Read the model definition and answer for the solid it produces. Units are mm, in the model's axes. A direction names the side the tool comes from. Coordinates: 2 decimals unless noted, no trailing zeros. Loops run counter-clockwise (first coordinate to the right, second up) from the corner with the lowest first, then second, coordinate; pieces in that order, holes last.
from build123d import *

# Parameters (mm, degrees)
F1_DEPTH = 29
F2_W     = 36
F2_H     = 11
F3_DEPTH = 127.001
F5_DEPTH = 58.001
F7_DEPTH = 58.001
F9_DEPTH = 33.001


with BuildPart() as f1:
    # F0 (on Front) → F1 (new body, symmetric)
    with BuildSketch(Plane.XZ):
        Polygon((11, 6), (11, 0), (116, 0), (116, 6), (127, 6), (127, 44), (0, 44), (0, 6), align=None)
    extrude(amount=F1_DEPTH, both=True)

    # F2 (on face) → F3 (cut, through all)
    with BuildSketch(Plane.YZ.offset(127)):
        with Locations((0, 38.5)):
            Rectangle(F2_W, F2_H)
    extrude(amount=-F3_DEPTH, mode=Mode.SUBTRACT)

    # F4 (on face) → F5 (cut, through all)
    with BuildSketch(Plane.XZ.offset(29)):
        with BuildLine():
            ThreePointArc((0, 15), (8.493903, 35.506097), (29, 44))
            Line((29, 44), (0, 44))
            Line((0, 44), (0, 15))
        make_face()
    extrude(amount=-F5_DEPTH, mode=Mode.SUBTRACT)

    # F6 (on face) → F7 (cut, through all)
    with BuildSketch(Plane.XZ.offset(29)):
        with BuildLine():
            ThreePointArc((98, 44), (118.506097, 35.506097), (127, 15))
            Line((127, 15), (127, 44))
            Line((127, 44), (98, 44))
        make_face()
    extrude(amount=-F7_DEPTH, mode=Mode.SUBTRACT)

    # F8 (on face) → F9 (cut, through all)
    with BuildSketch(Plane.XY.offset(33)):
        with BuildLine():
            Line((102, 4.898486), (83, 4.898486))
            ThreePointArc((83, 4.898486), (78.101514, 0), (83, -4.898486))
            Line((83, -4.898486), (102, -4.898486))
            ThreePointArc((102, -4.898486), (106.898486, 0), (102, 4.898486))
        make_face()
        with BuildLine():
            Line((44, 4.898486), (25, 4.898486))
            ThreePointArc((25, 4.898486), (20.101514, 0), (25, -4.898486))
            Line((25, -4.898486), (44, -4.898486))
            ThreePointArc((44, -4.898486), (48.898486, 0), (44, 4.898486))
        make_face()
    extrude(amount=-F9_DEPTH, mode=Mode.SUBTRACT)


solid = f1.part
Item 1: A cutting plane is placed at C-C on y = 0. Determine the outline of the cut face in (x, z).
Numbers:
outline: (0, 6) - (11, 6) - (11, 0) - (20.1, 0) - (20.1, 33) - (6.26, 33) arc R29 ccw to (0, 15) - close; (48.9, 0) - (78.1, 0) - (78.1, 33) - (48.9, 33) - close; (106.9, 0) - (116, 0) - (116, 6) - (127, 6) - (127, 15) arc R29 ccw to (120.74, 33) - (106.9, 33) - close
Item 2: A cutting plane is placed at D-D on y = 15.5. Determine the outline of the cut face in (x, z).
Numbers:
outline: (0, 6) - (11, 6) - (11, 0) - (116, 0) - (116, 6) - (127, 6) - (127, 15) arc R29 ccw to (120.74, 33) - (6.26, 33) arc R29 ccw to (0, 15) - close
Item 3: Which of the six approach directions +Z, -Z, +X, -X, +Y, -Y give full straight-line access (tool end or side, diameter ignored) to faces 4 (the face through (116, 0, 3)), 5 (the face through (64, -18, 38)), 6 (the face through (5, 0, 6)), 7 (the face through (92, -4.898, 17))?
Numbers:
face 4: -Z, +X, +Y, -Y
face 5: +Z, +X, -X
face 6: -Z, -X, +Y, -Y
face 7: +Z, -Z
Item 4: A cutting plane is placed at A-A on z = 12.5. Determine the outline of the cut face in (x, y), then the cut area to 3 significant figures.
Numbers:
outline: (0, -29) - (127, -29) - (127, 29) - (0, 29) - close; hole (25, -4.9) - (44, -4.9) arc R4.9 ccw to (44, 4.9) - (25, 4.9) arc R4.9 ccw to start; hole (83, -4.9) - (102, -4.9) arc R4.9 ccw to (102, 4.9) - (83, 4.9) arc R4.9 ccw to start
area: 6,840 mm2
Item 5: Given pin 1 (1 mm diameter, centred on y = -19, z = 34.5, fed in from +X); pin 2 (1 mm diameter, centred on y = 22, z = 28.5, fed in from -X); pin 3 (3.5 mm diameter, centred on x = 7.5, y = 1, fed in from -Z), each flat-ended and moving along its own axis, determine where each tip first touches the part or whether it passes through.
Numbers:
pin 1: stops at x = 119.91
pin 2: stops at x = 3.08
pin 3: stops at z = 6
Item 6: A cutting plane is placed at B-B on x = 96. Determine the outline of the cut face in (y, z).
Numbers:
outline: (-29, 0) - (-4.9, 0) - (-4.9, 33) - (-18, 33) - (-18, 44) - (-29, 44) - close; (4.9, 0) - (29, 0) - (29, 44) - (18, 44) - (18, 33) - (4.9, 33) - close
Item 7: Find the intervals of material crossed by line 1 along Y through (x, z) = (84, 10); line 2 along Y through (x, z) = (25.5, 38); line 3 along X through (y, z) = (3.5, 16), in increasing order.
Numbers:
line 1: y = -29 to -4.9, 4.9 to 29
line 2: y = -29 to -18, 18 to 29
line 3: x = 0.02 to 21.57, 47.43 to 79.57, 105.43 to 126.98
Item 8: Determine the mould class of faces 1 (the face through (20.103, 0.108, 16.731)), 2 (the face through (64, 0, 33)), 3 (the face through (11, 0, 3)) for opening direction X: released by +X, released by -X, zero draft, split by the parting line, or undercut.
Numbers:
face 1: undercut
face 2: zero draft
face 3: released by -X
